CAD build for the part. Positions are in the model's coordinates, mm. A direction names the side the tool comes from. Give positions to 0.01 mm unless a question says otherwise; leave off trailing zeros. Write each loop counter-clockwise with the first axis right and the second up, starting at its lowest first coordinate (ties: lowest second). Pieces come first, ordered by that corner, then holes. Notation, with made-up numbers: M -7,14.25 L 32,14.25 A28 ccw 32,37.25 Z; hole C 7,37.25 d1. An arc over 180 degrees is marked long. One line per question, with ' | ' between items. Start each with the question number.
1. Pull direction X, two halves, no side cores. Call faces 1 (the face through (1.5, 11.07, -52.53)), 2 (the face through (19, 0, -17)), 3 (the face through (18, 4, -32.738)), 4 (the face through (12, 12.5, -53)): released by +X, released by -X, zero draft, split by the parting line, or undercut.
2. Which spindle directions (+Z, -Z, +X, -X, +Y, -Y) get a long thin tool onto all of the face, cutting with end or side? Do faces 5 (the face through (2.958, -9.427, -9.055)), 6 (the face through (12, -12.5, -53)), 7 (the face through (23.57, -11, -52.95)), 8 (the face through (1.43, -11, -52.95)). Say none if no direction does.
3. Cut at A-A, the plane y = 0. Write the cut outline in (x, z).
4. Cut at B-B, the plane x = 12.5. Write the cut outline in (y, z).
5. Cut at D-D, the plane z = -35. Write the cut outline in (x, y).
6. Wall check: L1, parallel to X at y = -4, z = -9.5; L2, parallel to Y at x = 12.5, z = -58.5; L3, parallel to Z at x = 3.35, y = 0. Give the ranges that are in metal, low to high.
7. Flat gauge pins, fed straight in: pin 1 (7.5 mm diameter, centred on x = 9, z = -59, fed in from -Y); pin 2 (1 mm diameter, centred on x = 12, z = -47, fed in from +Y); pin 3 (3.5 mm diameter, centred on y = 0, z = -21.74, fed in from -X). Where does each tip first touch, or does it go through?
8. Cut at C-C, the plane z = -43.5. Write the cut outline in (x, y), then the cut area to 3 significant figures.
```python
from build123d import *

# Parameters (mm, degrees)
SKETCH1_R           = 3
BOSS_EXTRUDE1_DEPTH = 25
SKETCH3_R           = 6.4
CUT_EXTRUDE2_DEPTH  = 108
SKETCH4_W           = 13
SKETCH4_H           = 40.487648952
CUT_EXTRUDE3_DEPTH  = 25
FILLET2_R           = 5
SKETCH5_OUTSIDE_W   = 41.764
SKETCH5_OUTSIDE_H   = 51.764
SKETCH5_OUTSIDE_R   = 17.5
CUT_EXTRUDE5_DEPTH  = 39


with BuildPart() as part:
    # Sketch1 → Boss-Extrude1 (new body)
    with BuildSketch(Plane(origin=(0, 0, 0), x_dir=(0, 0, -1), z_dir=(1, 0, 0))):
        with BuildLine():
            Line((67.738148954, 12.5), (37.738148954, 12.5))
            Line((37.738148954, 12.5), (37.738148954, 17.5))
            Line((37.738148954, 17.5), (21.738148954, 17.5))
            ThreePointArc((21.738148954, 17.5), (11.838654018, 13.399494937), (7.738148954, 3.5))
            Line((7.738148954, 3.5), (7.738148954, -3.5))
            ThreePointArc((7.738148954, -3.5), (11.838654018, -13.399494937), (21.738148954, -17.5))
            Line((21.738148954, -17.5), (37.738148954, -17.5))
            Line((37.738148954, -17.5), (37.738148954, -12.5))
            Line((37.738148954, -12.5), (67.738148954, -12.5))
            Line((67.738148954, -12.5), (67.738148954, 12.5))
        make_face()
        with Locations((21.738148954, 0)):
            Circle(SKETCH1_R, mode=Mode.SUBTRACT)
    extrude(amount=BOSS_EXTRUDE1_DEPTH)

    # Sketch3 → Cut-Extrude2 (cut)
    with BuildSketch(Plane(origin=(0, 0, -67.738148954), x_dir=(-1, 0, 0), z_dir=(0, 0, -1))):
        with Locations((-12.5, 0)):
            Circle(SKETCH3_R)
    extrude(amount=-CUT_EXTRUDE2_DEPTH, mode=Mode.SUBTRACT)

    # Sketch4 → Cut-Extrude3 (cut)
    with BuildSketch(Plane.XY.offset(-7.738148954)):
        with Locations((12.5, 0)):
            Rectangle(SKETCH4_W, SKETCH4_H)
    extrude(amount=-CUT_EXTRUDE3_DEPTH, mode=Mode.SUBTRACT)

    # Fillet2
    fillet2_edges = [part.edges().sort_by_distance(p)[0] for p in [
        (0, 12.5, -52.738148954),
        (25, -12.5, -52.738148954),
        (25, 12.5, -52.738148954),
        (0, -12.5, -52.738148954),
    ]]
    fillet(fillet2_edges, radius=FILLET2_R)

    # Sketch5 outside → Cut-Extrude5 (cut)
    with BuildSketch(Plane(origin=(0, 0, -37.738148954), x_dir=(-1, 0, 0), z_dir=(0, 0, -1))):
        with Locations((-12.5, 0)):
            Rectangle(SKETCH5_OUTSIDE_W, SKETCH5_OUTSIDE_H)
        with Locations((-12.5, 0)):
            Circle(SKETCH5_OUTSIDE_R, mode=Mode.SUBTRACT)
    extrude(amount=-CUT_EXTRUDE5_DEPTH, mode=Mode.SUBTRACT)


solid = part.part
```
Here are the results:
1) face 1: released by -X | face 2: undercut | face 3: undercut | face 4: zero draft
2) face 5: +Z, +X, -X, -Y | face 6: -Z, +X, -X, -Y | face 7: -Z, +X, -Y | face 8: -Z, -X, -Y
3) outline: M 0,-67.74 L 6.1,-67.74 L 6.1,-32.74 L 6,-32.74 L 6,-24.74 L 0,-24.74 Z; M 0,-18.74 L 6,-18.74 L 6,-7.74 L 0,-7.74 Z; M 18.9,-67.74 L 25,-67.74 L 25,-24.74 L 19,-24.74 L 19,-32.74 L 18.9,-32.74 Z; M 19,-18.74 L 25,-18.74 L 25,-7.74 L 19,-7.74 Z
4) outline: M -17.5,-37.74 L -12.5,-37.74 L -12.5,-67.74 L -6.4,-67.74 L -6.4,-32.74 L -17.5,-32.74 Z; M 6.4,-67.74 L 12.5,-67.74 L 12.5,-37.74 L 17.5,-37.74 L 17.5,-32.74 L 6.4,-32.74 Z
5) outline: M 0,-12.25 A17.5 ccw 25,-12.25 L 25,12.25 A17.5 ccw 0,12.25 Z; hole C 12.5,0 d12.8
6) L1: 0 to 6, 19 to 25 | L2: -12.5 to -6.4, 6.4 to 12.5 | L3: -67.74 to -24.74, -18.74 to -7.74
7) pin 1: y = -12.5 | pin 2: y = 12.5 | pin 3: through
8) outline: M 0,-7.5 A5 ccw 5,-12.5 L 20,-12.5 A5 ccw 25,-7.5 L 25,7.5 A5 ccw 20,12.5 L 5,12.5 A5 ccw 0,7.5 Z; hole C 12.5,0 d12.8 | area: 475 mm^2
